Verification items for the finished model (mm, model axes). A direction names the side the tool comes from. Coordinates: 2 decimals unless noted, no trailing zeros. Order: outer loops, then holes, each group sorted by start corner. A loop starts at its lowest first (then second) coordinate and runs counter-clockwise, first axis right, second up. Notation, with made-up numbers: (74.25, -23.5) -> (101.25, -23.5) arc R32 ccw to (101.25, 11.5) -> close; hole circle Ø7 at (9, -13.5). An arc over 180 degrees is marked (long way). Write each question's results on one line, items separated by ' | '. Start each with the question number.
(1) Thickness scan on probe 1 along X at (y, z) = (-2, 40); probe 2 along Z at (x, y) = (-24.5, -24); probe 3 along X at (y, z) = (23, -20). Record the ranges inside material, lowest first. Write a range as [from, to].
(2) Set-up check for faces 5 (the flat face through (-13.472, -10, -7)), 6 (the flat face through (15.478, -33, -12)), 7 (the flat face through (-5, 27, 0)): record each of +Z, -Z, +X, -X, +Y, -Y from which the full face is reachable in a straight line by a thin tool's end or side.
(3) Cross-section at B-B on x = 35. Enter the section's corners in (y, z).
(4) Cross-section at A-A on x = -15.5. Enter the section's corners in (y, z), and give its area (3 significant figures).
(5) Go/stop test with flat-tipped pins: pin 1 (6 mm diameter, centred on x = 15.5, z = -27.5, fed in from +Y); pin 2 (11.5 mm diameter, centred on x = -13, z = 34.5, fed in from +Y); pin 3 (11.5 mm diameter, centred on x = -14, y = 25, fed in from +Z). Record where each tip stops, or that it passes through.
(6) Draft check along Y on faces 1 (the cylindrical face through (30.268, -22.211, -23.726)), 2 (the flat face through (-4.522, -22, -34)), 3 (the cylindrical face through (-4.13, -8.76, -8.2)), 4 (the flat face through (-5, 0, 27)). Enter one of: +Y half, -Y half, draft (parallel to the pull), parting line (faces both ways), or undercut.
```python
from build123d import *

# Parameters (mm, degrees)
REVOLVE1_ANGLE = 270


with BuildPart() as part:
    # Sketch2 → Revolve1 (revolve)
    with BuildSketch(Plane.XY):
        Polygon((-54.522496773, 27), (-54.522496773, 0), (45.477503227, 0), (45.477503227, 32.5), (15.477503227, 32.5), (15.477503227, 50), (-4.522496773, 50), (-4.522496773, 40), (-18.80529032, 40), align=None)
    revolve(axis=Axis((88.99, 0, 0), (-1, 0, 0)), revolution_arc=REVOLVE1_ANGLE)

    # Sketch3 → Cut-Revolve1 (revolve, cut)
    with BuildSketch(Plane.XY):
        Polygon((-54.522496773, 0), (45.477503227, 0), (45.477503227, 22.717967697), (5.477503227, 12), (-13.471731936, 12), (-13.471731936, 17), (-54.522496773, 17), align=None)
    revolve(axis=Axis((-54.522496773, 0, 0), (1, 0, 0)), mode=Mode.SUBTRACT)


solid = part.part
```
Results are:
1) probe 1: x = [-4.52, 15.48] | probe 2: z = [-29.37, 29.37] | probe 3: x = [-44.96, 45.48]
2) face 5: -X | face 6: +X | face 7: +Z, +X, -X, +Y
3) outline: (0, 19.91) -> (0, 32.5) arc R32.5 ccw (long way) to (32.5, 0) -> (19.91, 0) arc R19.91 cw (long way) to start
4) outline: (0, 17) -> (0, 40) arc R40 ccw (long way) to (40, 0) -> (17, 0) arc R17 cw (long way) to start | area: 3,090 mm2
5) pin 1: stops at y = 43.59 | pin 2: stops at y = 0 | pin 3: stops at z = 0
6) face 1: parting line | face 2: draft | face 3: undercut | face 4: +Y half
